```python
from build123d import *

# Parameters (mm, degrees)
SKETCH1_W               = 100
SKETCH1_H               = 50
BOSS_EXTRUDE1_DEPTH     = 10
SKETCH2_W               = 70
SKETCH2_H               = 5.887144663
BOSS_EXTRUDE2_DEPTH     = 60
SKETCH3_R               = 3
CUT_EXTRUDE1_DEPTH      = 10
CUT_EXTRUDE1_DEPTH_BACK = 10
FILLET1_R               = 2
FILLET2_R               = 2
FILLET3_R               = 2
FILLET4_R               = 2
FILLET5_R               = 2


with BuildPart() as part:
    # Sketch1 → Boss-Extrude1 (new body)
    with BuildSketch(Plane(origin=(0, 0, 0), x_dir=(1, 0, 0), z_dir=(0, 1, 0))):
        with Locations((6.899810964, -1.748582231)):
            Rectangle(SKETCH1_W, SKETCH1_H)
    extrude(amount=BOSS_EXTRUDE1_DEPTH)

    # Sketch2 → Boss-Extrude2 (add)
    with BuildSketch(Plane(origin=(0, 0, 0), x_dir=(1, 0, 0), z_dir=(0, 1, 0))):
        with Locations((21.899810964, -1.748582231)):
            Rectangle(SKETCH2_W, SKETCH2_H)
    extrude(amount=BOSS_EXTRUDE2_DEPTH)

    # Sketch3 → Cut-Extrude1 (cut, two sides)
    with BuildSketch(Plane.XY.offset(4.692154562)) as cut_extrude1_sk:
        with Locations(Location((4.078525913, 45.713993349, 0), (0, 0, 180))):  # turned: the seam where the file's is
            Circle(SKETCH3_R)
        with Locations(Location((41.437726316, 45.713993349, 0), (0, 0, 180))):  # turned: the seam where the file's is
            Circle(SKETCH3_R)
    extrude(amount=CUT_EXTRUDE1_DEPTH, mode=Mode.SUBTRACT)
    extrude(cut_extrude1_sk.sketch, amount=-CUT_EXTRUDE1_DEPTH_BACK, mode=Mode.SUBTRACT)

    # Fillet1
    fillet1_edges = [part.edges().sort_by_distance(p)[0] for p in [
        (21.899810964, 60, 4.692154562),
    ]]
    fillet(fillet1_edges, radius=FILLET1_R)

    # Fillet2
    fillet2_edges = [part.edges().sort_by_distance(p)[0] for p in [
        (21.899810964, 60, -1.194990101),
    ]]
    fillet(fillet2_edges, radius=FILLET2_R)

    # Fillet3
    fillet3_edges = [part.edges().sort_by_distance(p)[0] for p in [
        (21.899810964, 10, -1.194990101),
    ]]
    fillet(fillet3_edges, radius=FILLET3_R)

    # Fillet4
    fillet4_edges = [part.edges().sort_by_distance(p)[0] for p in [
        (21.899810964, 10, 4.692154562),
    ]]
    fillet(fillet4_edges, radius=FILLET4_R)

    # Fillet5
    fillet5_edges = [part.edges().sort_by_distance(p)[0] for p in [
        (-13.100189036, 10, 1.748582231),
    ]]
    fillet(fillet5_edges, radius=FILLET5_R)


solid = part.part
```
Source: CAD feature listing. Evaluate the final solid. Frame: model axes, mm. A direction names the side the tool comes from. Coordinates: 2 decimals unless noted, no trailing zeros. Write each loop counter-clockwise with the first axis right and the second up, starting at its lowest first coordinate (ties: lowest second). Pieces come first, ordered by that corner, then holes. Notation, with made-up numbers: (-19.75, 56) -> (24.25, 56) arc R9 cw to (24.25, 64) -> close; hole circle Ø1 at (54.25, 79.25). An arc over 180 degrees is marked (long way). Return JSON: item names as keys, results as strings. Group by question number.
1) Mould query, pull axis X, two halves, no side actions, for faces 3 (the face through (4.729, 48.643, 1.79)), 4 (the face through (42.088, 48.643, 1.79)), 5 (the face through (21, 35, 4.692)), 6 (the face through (-13.1, 36, 2)). Classes: +X half, -X half, draft (parallel to the pull), parting line (faces both ways), or undercut.
2) Set-up query: faces 1 (the face through (20.396, 10.601, 5.262)), 2 (the face through (21, 35, -1.195)). Return all of +Z, -Z, +X, -X, +Y, -Y with unobstructed straight access to the full face (end or side cutting, diameter ignored); none if empty.
3) Section query A-A, the plane x = 35.5. Return loops of the section in (y, z) (3 decimals).
4) Section query B-B, the plane z = 20.5. Return loops of the section in (x, y), plus the area to 3 significant figures.
5) Ray query, line 1 along Y through (x, z) = (4, 0.5); line 2 along Y through (x, z) = (25.5, -21); line 3 along Z through (x, y) = (43, 12) (3 decimals). Return the intervals inside material, ascending.
6) Section query C-C, the plane y = 33.5. Return loops of the section in (x, z) (3 decimals), plus the area to 3 significant figures.
7) Contact query for flat-ended pins moving along their axis: P1, Ø14, axis at x = 4.5, y = 29, coming from the -Z side (3 decimals); P2, Ø1.5, axis at x = 38.5, y = 16.5, coming from the +Z side; P3, Ø3, axis at y = 36, z = 1, coming from the -X side; P4, Ø1, axis at x = -19.5, z = -15, coming from the -Y side. Output: stop coordinate, or through.
From the geometry:
{
 "1": {"face 3": "undercut", "face 4": "undercut", "face 5": "draft", "face 6": "-X half"},
 "2": {"face 1": "+Z, +X, -X, +Y", "face 2": "-Z, +X, -X, +Y"},
 "3": {"outline": "(0, -23.251) -> (10, -23.251) -> (10, -3.195) arc R2 cw to (12, -1.195) -> (58, -1.195) arc R2 ccw to (60, 0.805) -> (60, 2.692) arc R2 ccw to (58, 4.692) -> (12, 4.692) arc R2 cw to (10, 6.692) -> (10, 26.749) -> (0, 26.749) -> close"},
 "4": {"outline": "(-43.1, 0) -> (56.9, 0) -> (56.9, 10) -> (-43.1, 10) -> close", "area": "1,000 mm²"},
 "5": {"line 1": "0 to 42.72, 48.71 to 59.98", "line 2": "0 to 10", "line 3": "-1.195 to 4.692"},
 "6": {"outline": "(-13.1, -1.195) -> (56.9, -1.195) -> (56.9, 4.692) -> (-13.1, 4.692) -> close", "area": "412 mm²"},
 "7": {"P1": "z = -1.195", "P2": "z = 4.69", "P3": "x = -13.1", "P4": "y = 0"}
}
